Geometry check sheet. Reference: drawing and pictorial views, mm from the part's lowest x, y, z. Coordinates: 2 decimals unless noted, no trailing zeros. Loops run counter-clockwise (first coordinate to the right, second up) from the corner with the lowest first, then second, coordinate; pieces in that order, holes last. Notation, with made-up numbers: (-19, 88.25) -> (34, 88.25) arc R18 cw to (34, 93.25) -> close; hole circle Ø3 at (-37.75, 29.25). An arc over 180 degrees is marked (long way). Use one line per item in the form item = value.
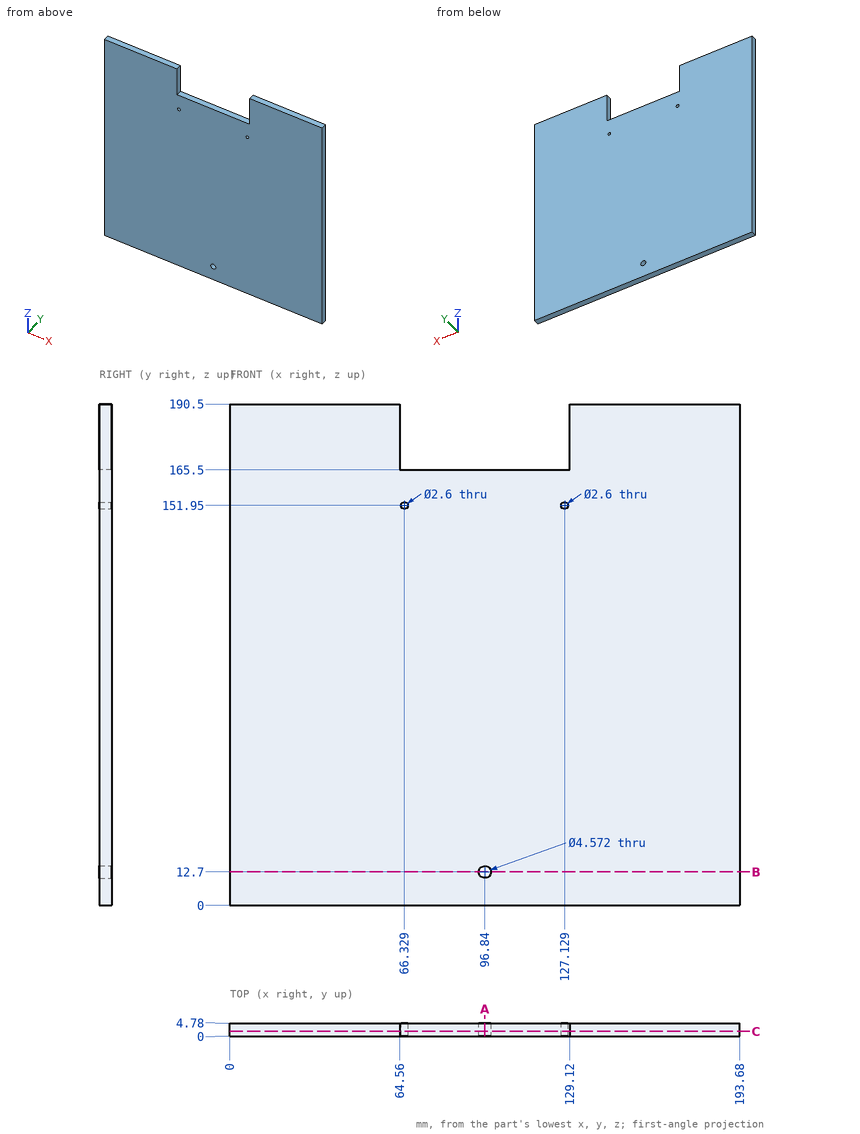
(1) Scan lines: line 1 along X through (y, z) = (1.05, 151.95); line 2 along Z through (x, y) = (96.84, 2.35); line 3 along X through (y, z) = (3, 172.5). Record each from-to range of solid material in increasing order.
Established:
line_1 = 0 to 65.03, 67.63 to 125.83, 128.43 to 193.68
line_2 = 0 to 10.41, 14.99 to 165.5
line_3 = 0 to 64.56, 129.12 to 193.68
(2) Section check A-A, the plane x = 96.84. Record the boundary of the cut face in (y, z).
Established:
outline = (0, 0) -> (4.78, 0) -> (4.78, 10.41) -> (0, 10.41) -> close; (0, 14.99) -> (4.78, 14.99) -> (4.78, 165.5) -> (0, 165.5) -> close
(3) Section check B-B, the plane z = 12.7. Record the boundary of the cut face in (x, y), plus the area to 3 significant figures.
Established:
outline = (0, 0) -> (94.55, 0) -> (94.55, 4.78) -> (0, 4.78) -> close; (99.13, 0) -> (193.68, 0) -> (193.68, 4.78) -> (99.13, 4.78) -> close
area = 904 mm²
(4) Section check C-C, the plane y = 1.8. Record the boundary of the cut face in (x, z).
Established:
outline = (0, 0) -> (193.68, 0) -> (193.68, 190.5) -> (129.12, 190.5) -> (129.12, 165.5) -> (64.56, 165.5) -> (64.56, 190.5) -> (0, 190.5) -> close; hole circle Ø2.6 at (66.33, 151.95); hole circle Ø4.57 at (96.84, 12.7); hole circle Ø2.6 at (127.13, 151.95)
(5) Go/stop test with flat-tipped pins: P1, Ø2.5, axis at x = 89, y = 3, coming from the +Z side; P2, Ø1.6, axis at x = 127.129, z = 151.95, coming from the +Y side. Record where each tip stops, or that it passes through.
Established:
P1 = 165.5
P2 = through
